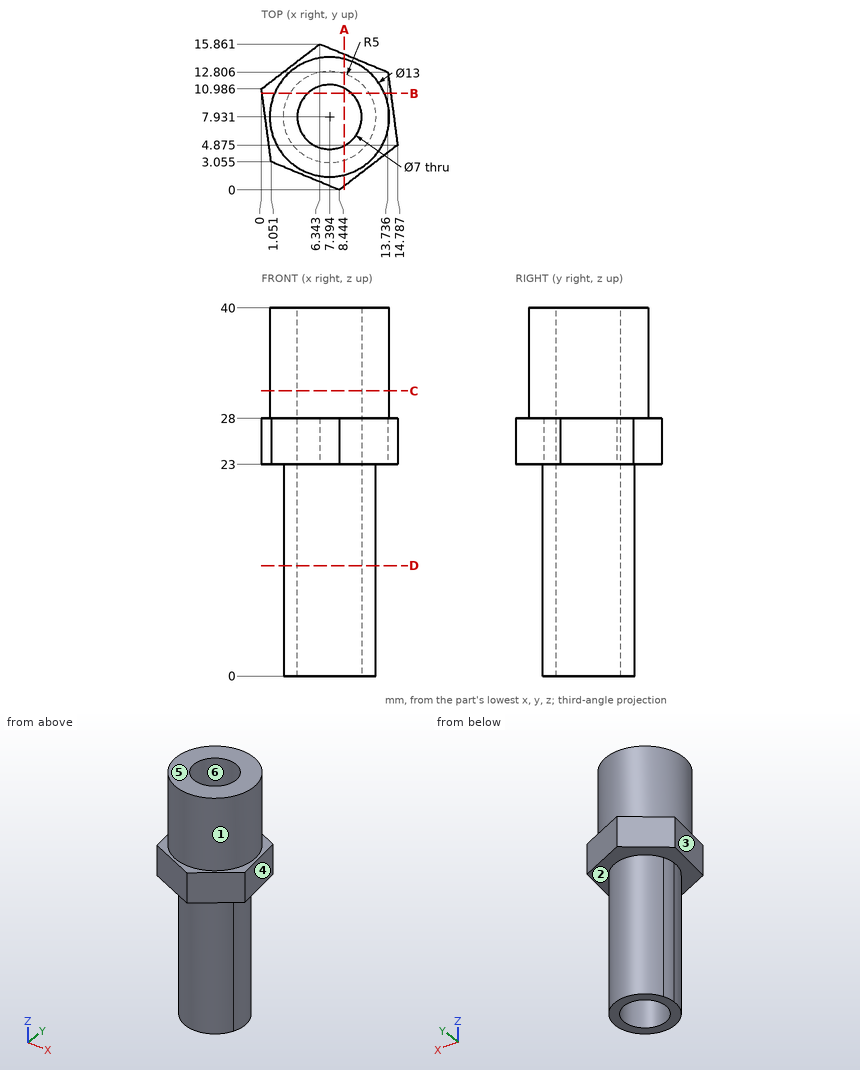
Answer from the drawing. Dimensions are ordinates in mm from the lowest x, y and z of the part. A direction names the side the tool comes from. Round coordinates to 2 decimals unless told otherwise and drop trailing zeros. Loops run counter-clockwise (first coordinate to the right, second up) from the corner with the lowest first, then second, coordinate; pieces in that order, holes last.
1) Given P1, Ø8, axis at x = 4.5, z = 35.5, coming from the +Y side; P2, Ø1.5, axis at x = 9, z = 7.5, coming from the -Y side (1 decimal); P3, Ø3, axis at x = 10, z = 4, coming from the +Y side, each flat-ended and moving along its own axis, determine where each tip first touches the part or whether it passes through.
Outcome:
P1: stops at y = 14.43
P2: stops at y = 3
P3: stops at y = 12.81
2) For the marked faces 1, 2 and 3, determine the directions among +Z, -Z, +X, -X, +Y, -Y from which every point of the face is accessible in a straight line to the end or side of a thin tool.
Outcome:
face 1: +Z
face 2: -Z
face 3: +Z, -Z, -X, -Y
3) A cutting plane is placed at B-B on y = 10.5. Determine the outline of the cut face in (x, z) (1 decimal).
Outcome:
outline: (0.1, 23) - (3.1, 23) - (3.1, 0) - (5, 0) - (5, 40) - (1.4, 40) - (1.4, 28) - (0.1, 28) - close; (9.8, 0) - (11.7, 0) - (11.7, 23) - (14, 23) - (14, 28) - (13.4, 28) - (13.4, 40) - (9.8, 40) - close
4) A cutting plane is placed at C-C on z = 31. Determine the outline of the cut face in (x, y).
Outcome:
outline: circle Ø13 at (7.39, 7.93); hole circle Ø7 at (7.39, 7.93)
5) A cutting plane is placed at A-A on x = 9. Determine the outline of the cut face in (y, z) (1 decimal).
Outcome:
outline: (0.4, 23) - (3.2, 23) - (3.2, 0) - (4.8, 0) - (4.8, 40) - (1.6, 40) - (1.6, 28) - (0.4, 28) - close; (11, 0) - (12.7, 0) - (12.7, 23) - (14.8, 23) - (14.8, 28) - (14.2, 28) - (14.2, 40) - (11, 40) - close
6) Consider line 1 (Y direction, x = 4.5, z = 26) (1 decimal); line 2 (Z direction, x = 2, y = 7.5); line 3 (X direction, y = 9.5, z = 35.5) (1 decimal). Determine where each line is inside the solid, lowest interval first.
Outcome:
line 1: y = 1.6 to 6, 9.9 to 14.4
line 2: z = 23 to 40
line 3: x = 1.1 to 4.3, 10.5 to 13.7
7) For a pull along X with two mould halves and no side action, classify the marked faces 4, 5 and 6 as released by +X, released by -X, zero draft, split by the parting line, or undercut.
Outcome:
face 4: released by +X
face 5: zero draft
face 6: undercut
8) A cutting plane is placed at D-D on z = 12. Determine the outline of the cut face in (x, y) (1 decimal).
Outcome:
outline: circle Ø10 at (7.4, 7.9); hole circle Ø7 at (7.4, 7.9)
